```python
from build123d import *

# Parameters (mm, degrees)
F0_R     = 25.4
F1_DEPTH = 6.35
F3_DEPTH = 12.7
F5_COUNT = 6
F6_R     = 6.35
F7_DEPTH = 25.4


with BuildPart() as f1:
    # F0 (on Right) → F1 (new body, symmetric)
    with BuildSketch(Plane.YZ):
        Circle(F0_R)
    extrude(amount=F1_DEPTH, both=True)

    # F2 (on face) → F3 (join)
    with BuildSketch(Plane.YZ.offset(6.35)):
        Polygon((-6.574004, 24.534516), (0, 0), (0, 24.534516), align=None)
        Polygon((0, 24.534516), (0, 0), (6.574004, 24.534516), align=None)
        Polygon((-6.574004, 24.534516), (0, 24.534516), (6.574004, 24.534516), (6.631173, 34.694516), (-6.574004, 34.694516), align=None)
    extrude(amount=-F3_DEPTH)

    # F5: F1 ×6 about axis
    f5_axis = Axis((-31.581827, 0, 0), (-1, 0, 0))


with BuildPart() as f1_1:
    add(f1.part)
    for i in range(1, F5_COUNT):
        add(f1.part.rotate(f5_axis, i * 360 / F5_COUNT))

    # F6 (on face) → F7 (cut)
    with BuildSketch(Plane.YZ.offset(6.35)):
        Circle(F6_R)
    extrude(amount=-F7_DEPTH, mode=Mode.SUBTRACT)


solid = f1_1.part
```
Geometry check sheet. Reference: the model listing, model coordinates, mm. A direction names the side the tool comes from. Coordinates: 2 decimals unless noted, no trailing zeros. Loops run counter-clockwise (first coordinate to the right, second up) from the corner with the lowest first, then second, coordinate; pieces in that order, holes last.
Item 1: Access from +Z, -Z, +X, -X, +Y, -Y to the whole of each face (thin tool, end or side, straight path). Record for faces 4 (the face through (0, -6.574, 30)), 5 (the face through (0.089, 22.422, 20.536)), 6 (the face through (6.35, -8, 0)).
Item 2: Sectioned sample at A-A, the plane z = 0. Record the boundary of the cut face in (x, y), then the cut area to 3 significant figures.
Item 3: Release check for a two-part mould opening along Y. For faces 1 (the face through (0.1, -25.4, 0.1)), 2 (the face through (0.089, -22.422, -20.536)), 3 (the face through (0, 0, 34.695)) record: released by +Y, released by -Y, zero draft, split by the parting line, or undercut.
Item 4: Thickness scan on line 1 (Z direction, x = 2.75, y = 0.5); line 2 (Y direction, x = -1.75, z = -21.5); line 3 (Z direction, x = 0.5, y = 3.5). Record the ranges inside material, lowest first.
Item 5: Sectioned sample at C-C, the plane x = 0.5. Record the boundary of the cut face in (y, z), then the cut area to 3 significant figures.
Item 6: Sectioned sample at D-D, the plane z = -19.5. Record the boundary of the cut face in (x, y), then the cut area to 3 significant figures.
Item 7: Sectioned sample at B-B, the plane y = 0. Record the boundary of the cut face in (x, z).
Item 8: Go/stop test with flat-tipped pins: pin 1 Ø1.5 at (x, z) = (0, 1) entering from -Y; pin 2 Ø3 at (x, z) = (-2.5, 27.5) entering from -Y; pin 3 Ø5 at (x, y) = (4, 24) entering from -Z; pin 4 Ø7.5 at (y, z) = (0, 0) entering from +X. Record where each tip stops, or that it passes through.
Check result:
1. face 4: +Z, +X, -X, -Y
1. face 5: +Z, +X, -X
1. face 6: +Z, -Z, +X, +Y, -Y
2. outline: (-6.35, -25.4) - (6.35, -25.4) - (6.35, -6.35) - (-6.35, -6.35) - close; (-6.35, 6.35) - (6.35, 6.35) - (6.35, 25.4) - (-6.35, 25.4) - close
2. area: 484 mm2
3. face 1: released by -Y
3. face 2: undercut
3. face 3: zero draft
4. line 1: z = -34.69 to -6.33, 6.33 to 34.69
4. line 2: y = -27.65 to -24.09, -13.52 to 13.52, 24.01 to 27.65
4. line 3: z = -34.69 to -5.3, 5.3 to 34.69
5. outline: (-33.36, -11.6) - (-26.76, -23.04) - (-17.96, -17.96) arc R25.4 ccw to (-6.57, -24.53) - (-6.63, -34.69) - (6.57, -34.69) - (6.57, -24.53) arc R25.4 ccw to (17.96, -17.96) - (26.73, -23.09) - (33.33, -11.65) - (24.53, -6.57) arc R25.4 ccw to (24.53, 6.57) - (33.36, 11.6) - (26.76, 23.04) - (17.96, 17.96) arc R25.4 ccw to (6.57, 24.53) - (6.63, 34.69) - (-6.57, 34.69) - (-6.57, 24.53) arc R25.4 ccw to (-17.96, 17.96) - (-26.73, 23.09) - (-33.33, 11.65) - (-24.53, 6.57) arc R25.4 ccw to (-24.53, -6.57) - close; hole circle Ø12.7 at (0, 0)
5. area: 2,660 mm2
6. outline: (-6.35, -28.8) - (6.35, -28.8) - (6.35, -20.63) - (-6.35, -20.63) - close; (-6.35, -16.28) - (6.35, -16.28) - (6.35, 16.28) - (-6.35, 16.28) - close; (-6.35, 20.59) - (6.35, 20.59) - (6.35, 28.8) - (-6.35, 28.8) - close
6. area: 622 mm2
7. outline: (-6.35, -34.69) - (6.35, -34.69) - (6.35, -6.35) - (-6.35, -6.35) - close; (-6.35, 6.35) - (6.35, 6.35) - (6.35, 34.69) - (-6.35, 34.69) - close
8. pin 1: stops at y = -25.4
8. pin 2: stops at y = -6.57
8. pin 3: stops at z = -22.96
8. pin 4: passes through
